Design review of the part built by this model. Coordinates are the model's own, in mm. Face numbers are marked on the shaded views. A direction names the side the tool comes from. Give positions to 0.01 mm unless a question says otherwise; leave off trailing zeros. Order: outer loops, then holes, each group sorted by start corner. A loop starts at its lowest first (then second) coordinate and runs counter-clockwise, first axis right, second up.
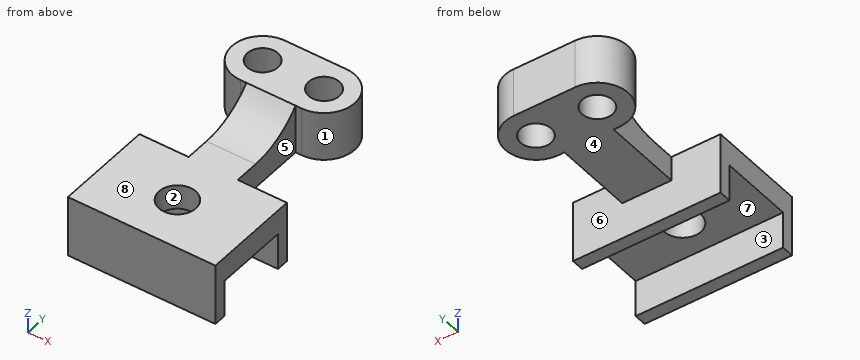
```python
from build123d import *

# Parameters (mm, degrees)
BOSS_EXTRUDE1_DEPTH     = 38.1
SKETCH2_R               = 9.525
CUT_EXTRUDE1_DEPTH      = 1
CUT_EXTRUDE1_DEPTH_BACK = 32.75
BOSS_EXTRUDE2_DEPTH     = 12.7
SKETCH4_R               = 7.9375
BOSS_EXTRUDE3_DEPTH     = 25.4


with BuildPart() as part:
    # Sketch1 → Boss-Extrude1 (new body, symmetric)
    with BuildSketch(Plane.YZ):
        Polygon((0, 0), (0, 31.75), (-50.8, 31.75), (-50.8, 0), (-44.45, 0), (-44.45, 19.05), (-6.35, 19.05), (-6.35, 0), align=None)
    extrude(amount=BOSS_EXTRUDE1_DEPTH, both=True)

    # Sketch2 → Cut-Extrude1 (cut, two sides)
    with BuildSketch(Plane.XY.offset(31.75)) as cut_extrude1_sk:
        with Locations((0, -25.4)):
            Circle(SKETCH2_R)
    extrude(amount=CUT_EXTRUDE1_DEPTH, mode=Mode.SUBTRACT)
    extrude(cut_extrude1_sk.sketch, amount=-CUT_EXTRUDE1_DEPTH_BACK, mode=Mode.SUBTRACT)

    # Sketch3 → Boss-Extrude2 (add, symmetric)
    with BuildSketch(Plane.YZ):
        with BuildLine():
            Line((0, 19.05), (41.098063314, 19.05))
            Line((41.098063314, 19.05), (41.098063314, 44.45))
            ThreePointArc((41.098063314, 44.45), (28.254259867, 35.069617598), (12.7, 31.75))
            Line((12.7, 31.75), (0, 31.75))
            Line((0, 31.75), (0, 19.05))
        make_face()
    extrude(amount=BOSS_EXTRUDE2_DEPTH, both=True)

    # Sketch4 → Boss-Extrude3 (add)
    with BuildSketch(Plane(origin=(0, 0, 19.05), x_dir=(1, 0, 0), z_dir=(0, 0, -1))):
        with BuildLine():
            Line((-15.875, -41.098063314), (15.875, -41.098063314))
            ThreePointArc((15.875, -41.098063314), (31.75, -56.973063314), (15.875, -72.848063314))
            Line((15.875, -72.848063314), (-15.875, -72.848063314))
            ThreePointArc((-15.875, -72.848063314), (-31.75, -56.973063314), (-15.875, -41.098063314))
        make_face()
        with Locations((15.875, -56.973063314)):
            Circle(SKETCH4_R, mode=Mode.SUBTRACT)
        with Locations((-15.875, -56.973063314)):
            Circle(SKETCH4_R, mode=Mode.SUBTRACT)
    extrude(amount=-BOSS_EXTRUDE3_DEPTH)


solid = part.part
```
1. For pin 1 (6 mm diameter, centred on x = 8, y = 7, fed in from +Z); pin 2 (10 mm diameter, centred on x = -11, y = -37, fed in from -Z); pin 3 (11.5 mm diameter, centred on x = 0, y = -25.4, fed in from +Z); pin 4 (21 mm diameter, centred on x = -13, z = 7, fed in from +Y), all flat-tipped, find the tip position at first contact; note any pin that passes through.
Recorded:
pin 1: stops at z = 31.75
pin 2: stops at z = 19.05
pin 3: passes through
pin 4: stops at y = 0
2. Take a section at C-C (y = 53). State the section outline as (x, z) points.
Recorded:
outline: (-31.24, 19.05) - (-22.75, 19.05) - (-22.75, 44.45) - (-31.24, 44.45) - close; (-9, 19.05) - (9, 19.05) - (9, 44.45) - (-9, 44.45) - close; (22.75, 19.05) - (31.24, 19.05) - (31.24, 44.45) - (22.75, 44.45) - close
3. Take a section at D-D (z = 24). State how many separate pieces and enclosed holes the cut face has, then the cut area to 3 significant figures.
Recorded:
separate pieces: 1
enclosed holes: 3
area: 6,030 mm2
4. Machinability: for the marked faces 4, 5, 6, 7 and 8, which of the approach directions +Z, -Z, +X, -X, +Y, -Y give a long, thin tool a straight path to every point of the face, cutting with its end or side? Answer none if there is none.
Recorded:
face 4: -Z, +X, -X, +Y
face 5: +Z, -Z, +X
face 6: -Z
face 7: -Z, +X, -X
face 8: +Z, +X, -X, -Y
5. Draft analysis for pull direction X (two halves, no side actions). For the marked faces 1, 2 and 3, state which applies: pulls with the +X half, pulls with the -X half, needs draft (parallel to the pull), parting line crosses it, or undercut.
Recorded:
face 1: pulls with the +X half
face 2: undercut
face 3: needs draft
6. Take a section at A-A (y = -25.4). State the section outline as (x, z) points (3 decimals), then the cut area to 3 significant figures.
Recorded:
outline: (-38.1, 19.05) - (-9.525, 19.05) - (-9.525, 31.75) - (-38.1, 31.75) - close; (9.525, 19.05) - (38.1, 19.05) - (38.1, 31.75) - (9.525, 31.75) - close
area: 726 mm2
7. Take a section at B-B (x = 0). State the section outline as (y, z) points (3 decimals), then the cut area to 3 significant figures.
Recorded:
outline: (-50.8, 0) - (-44.45, 0) - (-44.45, 19.05) - (-34.925, 19.05) - (-34.925, 31.75) - (-50.8, 31.75) - close; (-15.875, 19.05) - (-6.35, 19.05) - (-6.35, 0) - (0, 0) - (0, 19.05) - (72.848, 19.05) - (72.848, 44.45) - (41.098, 44.45) arc R38.1 cw to (12.7, 31.75) - (-15.875, 31.75) - close
area: 2,080 mm2
8. For line 1 along Y through (x, z) = (9.5, 18); line 2 along Y through (x, z) = (19.5, 20); line 3 along X through (y, z) = (-25, 22), list the stretches that pass through material, from the lowest coordinate up.
Recorded:
line 1: y = -50.8 to -44.45, -6.35 to 0
line 2: y = -50.8 to 0, 41.52 to 49.91, 64.03 to 72.43
line 3: x = -38.1 to -9.52, 9.52 to 38.1
